from build123d import *

# Parameters (mm, degrees)
SKETCH_W        = 4.72
SKETCH_H        = 5.2
PAD_DEPTH       = 10
POCKET_DEPTH    = 38.001
POCKET005_DEPTH = 6
SKETCH003_R     = 1.5
POCKET006_DEPTH = 5
FILLET_R        = 1.99


with BuildPart() as part:
    # Sketch → Pad (new body)
    with BuildSketch(Plane.XY):
        Polygon((-19, 19), (-19, -19), (19, -19), (19, 19), (17, 19), (17, 26.7), (6, 26.7), (6, 19), (-6, 19), (-6, 26.7), (-17, 26.7), (-17, 19), align=None)
        with Locations((-12.41, 21.6)):
            Rectangle(SKETCH_W, SKETCH_H, mode=Mode.SUBTRACT)
        with Locations((12.41, 21.6)):
            Rectangle(SKETCH_W, SKETCH_H, mode=Mode.SUBTRACT)
    extrude(amount=PAD_DEPTH)

    # Sketch001 (on Face3 of Pad) → Pocket (cut, through all)
    with BuildSketch(Plane.YZ.offset(19)):
        Polygon((26.7, 3), (26.7, 0), (0, 0), (5.7, 3), align=None)
    extrude(amount=-POCKET_DEPTH, mode=Mode.SUBTRACT)

    # Sketch002 (on Face6 of Pocket) → Pocket005 (cut)
    with BuildSketch(Plane.XY.offset(10)):
        Polygon((-9.25, -19), (9.25, -19), (9.25, 6.35), (6, 6.35), (6, 19), (-6, 19), (-6, 6.35), (-9.25, 6.35), align=None)
    extrude(amount=-POCKET005_DEPTH, mode=Mode.SUBTRACT)

    # Sketch003 → Pocket006 (cut)
    with BuildSketch(Plane.XY.offset(4)):
        with Locations((-5.25, -5.15)):
            Circle(SKETCH003_R)
        with Locations((5.25, -5.15)):
            Circle(SKETCH003_R)
    extrude(amount=-POCKET006_DEPTH, mode=Mode.SUBTRACT)

    # Fillet
    fillet_edges = [part.edges().sort_by_distance(p)[0] for p in [
        (17, 26.7, 6.5),
        (6, 26.7, 6.5),
        (-6, 26.7, 6.5),
        (-17, 26.7, 6.5),
        (-19, 19, 6.5),
        (19, 19, 6.5),
        (19, -19, 5),
        (-19, -19, 5),
    ]]
    fillet(fillet_edges, radius=FILLET_R)


solid = part.part
The model under review builds one solid part; all positions refer to its coordinate system, in mm. A direction names the side the tool comes from. Give positions to 0.01 mm unless a question says otherwise; leave off trailing zeros. Order: outer loops, then holes, each group sorted by start corner. A loop starts at its lowest first (then second) coordinate and runs counter-clockwise, first axis right, second up. Notation, with made-up numbers: M 34,50 L 43,50 A22 ccw 43,77 Z; hole C -5.75,-22.75 d7. An arc over 180 degrees is marked long. One line per question, with ' | ' between items. Start each with the question number.
1) Consider section C-C, the plane y = -5.15. Give the boundary of the cut face in (x, z).
2) Mouldability with a two-part tool opening along Y and no side actions: class faces 5 (the face through (0.27, 2.81, 1.48)), 6 (the face through (17, 22, 6)), 7 (the face through (-12, 24.2, 6)) as pulls with the +Y half, pulls with the -Y half, needs draft (parallel to the pull), parting line crosses it, or undercut.
3) Clearance check with flat-ended pins moving along their axes: P1, Ø1, axis at x = -8, z = 8, coming from the -Y side; P2, Ø2.5, axis at y = 20.5, z = 5, coming from the +X side; P3, Ø6, axis at x = -3, y = -5, coming from the +Z side. State where each tip first meets the part, or that it passes through.
4) Wall thickness on L1, parallel to X at y = 12.5, z = 4.25; L2, parallel to Y at x = 11, z = 6.75; L3, parallel to X at y = -12, z = 6: over which ranges is each line inside the solid? List them lowest first. Write a range as from..to.
5) Consider section A-A, the plane z = 5. State how many separate pieces and enclosed holes the cut face has, then the cut area to 3 significant figures.
6) For faces 1 (the face through (-14.77, 22, 6)), 2 (the face through (8, 6.35, 7)), 3 (the face through (-17, 22, 6)), 4 (the face through (0.1, 19, 3.5)), list the 3-axis set-ups (+Z, -Z, +X, -X, +Y, -Y) from which the entire face can be reached by the end or side of a thin tool; tool diameter is ignored.
7) Consider section B-B, the plane x = 5.25. Give the boundary of the cut face in (y, z).
8) Consider section D-D, the plane z = 1. Give the boundary of the cut face in (x, y).
Found:
1) outline: M -19,0 L -6.75,0 L -6.75,4 L -9.25,4 L -9.25,10 L -19,10 Z; M -3.75,0 L 3.75,0 L 3.75,4 L -3.75,4 Z; M 6.75,0 L 19,0 L 19,10 L 9.25,10 L 9.25,4 L 6.75,4 Z
2) face 5: pulls with the +Y half | face 6: needs draft | face 7: undercut
3) P1: stops at y = 6.35 | P2: stops at x = 17 | P3: stops at z = 4
4) L1: x = -19..-6, 6..19 | L2: y = -19..19, 24.2..26.7 | L3: x = -19..-9.25, 9.25..19
5) separate pieces: 2 | enclosed holes: 2 | area: 937 mm²
6) face 1: +Z, -Z | face 2: +Z, -Y | face 3: +Z, -Z, -X, +Y | face 4: +Z, -Z, +Y
7) outline: M -19,0 L -6.65,0 L -6.65,4 L -19,4 Z; M -3.65,0 L 0,0 L 5.7,3 L 19,3 L 19,4 L -3.65,4 Z
8) outline: M -19,-17.01 A1.99 ccw -17.01,-19 L 17.01,-19 A1.99 ccw 19,-17.01 L 19,1.9 L -19,1.9 Z; hole C -5.25,-5.15 d3; hole C 5.25,-5.15 d3
